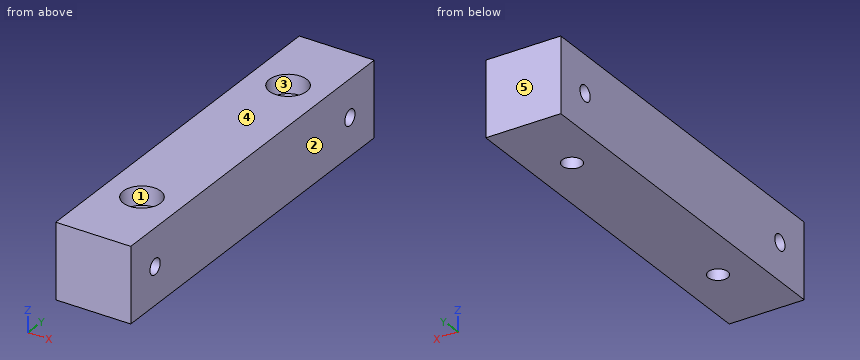
from build123d import *

# Parameters (mm, degrees)
F0_W     = 20
F0_H     = 100
F0_R     = 2.6
F1_DEPTH = 20
F2_R     = 5
F3_DEPTH = 5
F4_R     = 2.1
F5_DEPTH = 25


with BuildPart() as f1:
    # F0 (on Top) → F1 (new body)
    with BuildSketch(Plane.XY):
        Rectangle(F0_W, F0_H)
        with Locations((0, -30)):
            Circle(F0_R, mode=Mode.SUBTRACT)
        with Locations((0, 30)):
            Circle(F0_R, mode=Mode.SUBTRACT)
    extrude(amount=F1_DEPTH)

    # F2 (on face) → F3 (cut)
    with BuildSketch(Plane.XY.offset(20)):
        with Locations((0, 30)):
            Circle(F2_R)
        with Locations((0, -30)):
            Circle(F2_R)
    extrude(amount=-F3_DEPTH, mode=Mode.SUBTRACT)

    # F4 (on face) → F5 (cut)
    with BuildSketch(Plane.YZ.offset(10)):
        with Locations((-40, 10)):
            Circle(F4_R)
        with Locations((40, 10)):
            Circle(F4_R)
    extrude(amount=-F5_DEPTH, mode=Mode.SUBTRACT)


solid = f1.part
Design review of the part built by this model. Coordinates are the model's own, in mm. Face numbers are marked on the shaded views. A direction names the side the tool comes from. Give positions to 0.01 mm unless a question says otherwise; leave off trailing zeros. Loops run counter-clockwise (first coordinate to the right, second up) from the corner with the lowest first, then second, coordinate; pieces in that order, holes last. Notation, with made-up numbers: (80, 56.25) -> (128, 56.25) arc R16 ccw to (128, 61.25) -> close; hole circle Ø2 at (36.5, 83). An arc over 180 degrees is marked (long way). One line per question, with ' | ' between items. Start each with the question number.
(1) For line 1 (Y direction, x = 0, z = 16.4); line 2 (Z direction, x = -0.5, y = -40); line 3 (Y direction, x = 3.25, z = 18.75), list the stretches that pass through material, from the lowest coordinate up.
(2) We need section C-C (x = 4). State the section outline as (y, z) points.
(3) We need section A-A (x = 0). State the section outline as (y, z) points.
(4) Insertion check: P1, Ø8, axis at x = 0, y = -30.5, coming from the +Z side. The pin has a flat end and moves straight along its axis. Give the tip position at first contact, or say it passes through.
(5) Draft analysis for pull direction Y (two halves, no side actions). For the marked faces 3, 4 and 5, state which applies: +Y half, -Y half, draft (parallel to the pull), parting line (faces both ways), or undercut.
(6) We need section B-B (y = -30). State the section outline as (x, z) points, and give its area (3 significant figures).
(7) For the marked faces 1 and 2, list the 3-axis set-ups (+Z, -Z, +X, -X, +Y, -Y) from which the entire face can be reached by the end or side of a thin tool; tool diameter is ignored.
(8) We need section D-D (z = 17). State the section outline as (x, y) points, and give its area (3 significant figures).
The answers:
1) line 1: y = -50 to -35, -25 to 25, 35 to 50 | line 2: z = 0 to 7.9, 12.1 to 20 | line 3: y = -50 to -33.8, -26.2 to 26.2, 33.8 to 50
2) outline: (-50, 0) -> (50, 0) -> (50, 20) -> (33, 20) -> (33, 15) -> (27, 15) -> (27, 20) -> (-27, 20) -> (-27, 15) -> (-33, 15) -> (-33, 20) -> (-50, 20) -> close; hole circle Ø4.2 at (-40, 10); hole circle Ø4.2 at (40, 10)
3) outline: (-50, 0) -> (-32.6, 0) -> (-32.6, 15) -> (-35, 15) -> (-35, 20) -> (-50, 20) -> close; (-27.4, 0) -> (27.4, 0) -> (27.4, 15) -> (25, 15) -> (25, 20) -> (-25, 20) -> (-25, 15) -> (-27.4, 15) -> close; (32.6, 0) -> (50, 0) -> (50, 20) -> (35, 20) -> (35, 15) -> (32.6, 15) -> close; hole circle Ø4.2 at (-40, 10); hole circle Ø4.2 at (40, 10)
4) P1: stops at z = 15
5) face 3: undercut | face 4: draft | face 5: +Y half
6) outline: (-10, 0) -> (-2.6, 0) -> (-2.6, 15) -> (-5, 15) -> (-5, 20) -> (-10, 20) -> close; (2.6, 0) -> (10, 0) -> (10, 20) -> (5, 20) -> (5, 15) -> (2.6, 15) -> close | area: 272 mm^2
7) face 1: +Z | face 2: +Z, -Z, +X, +Y, -Y
8) outline: (-10, -50) -> (10, -50) -> (10, 50) -> (-10, 50) -> close; hole circle Ø10 at (0, -30); hole circle Ø10 at (0, 30) | area: 1,840 mm^2
